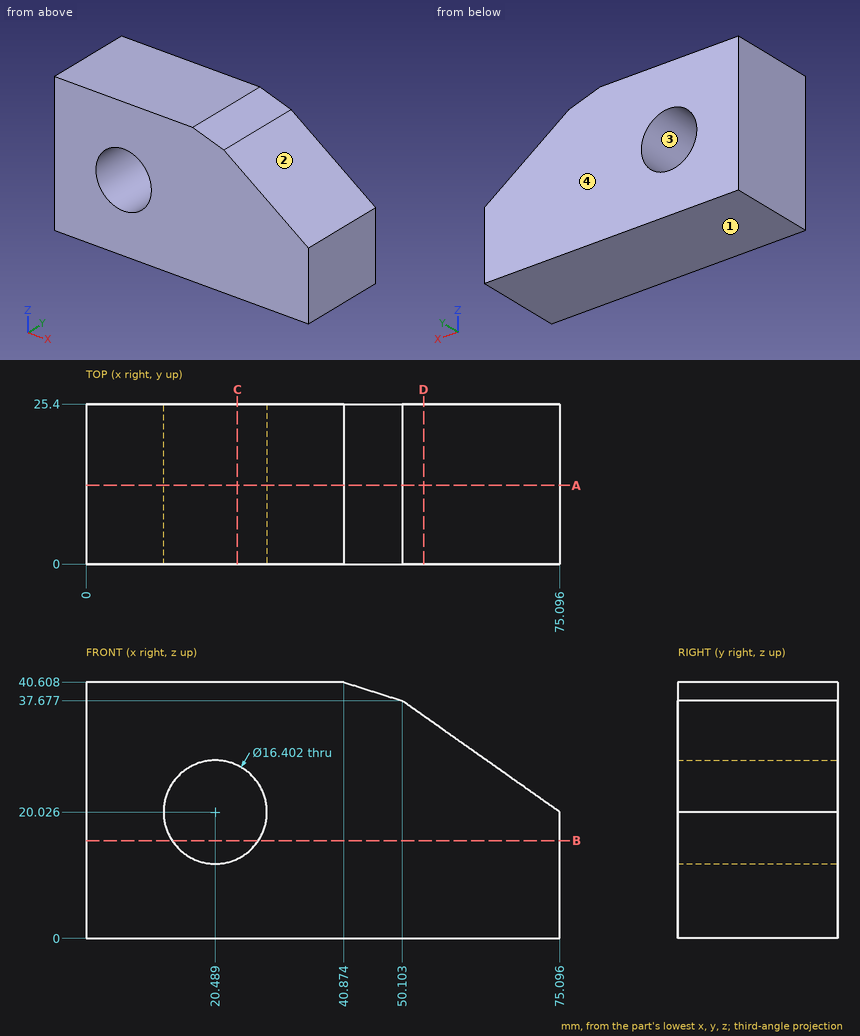
The drawing under review shows one solid part. Ordinate dimensions are in mm from its lowest x, y, z. Round coordinates to 2 decimals unless told otherwise and drop trailing zeros. Loops run counter-clockwise (first coordinate to the right, second up) from the corner with the lowest first, then second, coordinate; pieces in that order, holes last.
Item 1: Take a section at C-C (x = 24). Write out the cut boundary in (y, z).
Determined:
outline: (0, 0) - (25.4, 0) - (25.4, 12.61) - (0, 12.61) - close; (0, 27.44) - (25.4, 27.44) - (25.4, 40.61) - (0, 40.61) - close
Item 2: Take a section at B-B (z = 15.5). Write out the cut boundary in (x, y).
Determined:
outline: (0, 0) - (13.65, 0) - (13.65, 25.4) - (0, 25.4) - close; (27.33, 0) - (75.1, 0) - (75.1, 25.4) - (27.33, 25.4) - close
Item 3: For line 1 (X direction, y = 6.75, z = 19.5) (1 decimal); line 2 (Z direction, x = 15.5, y = 5) (1 decimal); line 3 (X direction, y = 6.5, z = 23) (1 decimal), list the stretches that pass through material, from the lowest coordinate up.
Determined:
line 1: x = 0 to 12.3, 28.7 to 75.1
line 2: z = 0 to 13.5, 26.5 to 40.6
line 3: x = 0 to 12.8, 28.1 to 70.9
Item 4: Mouldability with a two-part tool opening along Z and no side actions: class the marked faces 1, 2, 3 and 4 as released by +Z, released by -Z, zero draft, split by the parting line, or undercut.
Determined:
face 1: released by -Z
face 2: released by +Z
face 3: undercut
face 4: zero draft
Item 5: Take a section at D-D (x = 53.5). Write out the cut boundary in (y, z).
Determined:
outline: (0, 0) - (25.4, 0) - (25.4, 35.28) - (0, 35.28) - close
Item 6: Clearance check with flat-ended pins moving along their axes: pin 1 Ø4 at (x, y) = (59, 15.5) entering from +Z (1 decimal); pin 2 Ø8 at (y, z) = (9, 34) entering from +X (1 decimal). State where each tip first meets the part, or that it passes through.
Determined:
pin 1: stops at z = 32.8
pin 2: stops at x = 61
Item 7: Take a section at A-A (y = 12.5). Write out the cut boundary in (x, z) (1 decimal).
Determined:
outline: (0, 0) - (75.1, 0) - (75.1, 20) - (50.1, 37.7) - (40.9, 40.6) - (0, 40.6) - close; hole circle Ø16.4 at (20.5, 20)
